Work out the finished part from the listing and answer in its coordinate system (mm). A direction names the side the tool comes from. Give positions to 0.01 mm unless a question says otherwise; leave off trailing zeros. Loops run counter-clockwise (first coordinate to the right, second up) from the corner with the lowest first, then second, coordinate; pieces in that order, holes last. Notation, with made-up numbers: (83.25, -32) - (112.25, -32) arc R31 ccw to (112.25, 5) - close; hole circle Ø5 at (-10, 59). An arc over 180 degrees is marked (long way). One line per question, with ' | ' between items.
from build123d import *

# Parameters (mm, degrees)
SKIZZE1_W                                  = 70
SKIZZE1_H                                  = 20
AUFSATZ_LINEAR_AUSTRAGEN1_DEPTH            = 20
F_5_2_5_2_DURCHMESSER_BOHRUNG1_D           = 5.2
F_5_2_5_2_DURCHMESSER_BOHRUNG1_CSINK_D     = 5.25
F_5_2_5_2_DURCHMESSER_BOHRUNG1_CSINK_ANGLE = 90
SKIZZE21_R                                 = 6.05
SCHNITT_LINEAR_AUSTRAGEN3_DEPTH            = 7
SKIZZE22_R                                 = 4
SCHNITT_LINEAR_AUSTRAGEN5_DEPTH            = 10


# Read off the part's stored shape, not the designer's step: Durchgangsloch für M3.51
with BuildPart() as part:
    # Skizze1 → Aufsatz-Linear austragen1 (new body)
    with BuildSketch(Plane.XY):
        with Locations((0, 1.677024639)):
            Rectangle(SKIZZE1_W, SKIZZE1_H)
    extrude(amount=AUFSATZ_LINEAR_AUSTRAGEN1_DEPTH)

    # Ø5.2 (5.2) Durchmesser Bohrung1 (through all)
    with Locations(Plane.XY.offset(20)):
        with Locations((-28, 0.177024639), (28, 0.177024639)):
            CounterSinkHole(F_5_2_5_2_DURCHMESSER_BOHRUNG1_D / 2, F_5_2_5_2_DURCHMESSER_BOHRUNG1_CSINK_D / 2, counter_sink_angle=F_5_2_5_2_DURCHMESSER_BOHRUNG1_CSINK_ANGLE)

    # Durchgangsloch für M3.51 outline → Durchgangsloch für M3.51 (revolve, cut)
    with BuildSketch(Plane(origin=(-28, 0, 10), x_dir=(1, 0, 0), z_dir=(0, 0, 1))):
        Polygon((1.85, -8.297975361), (1.85, -1.649435315), (0, -1.649435315), (0, -8.322975361), (1.875, -8.322975361), align=None)
    revolve(axis=Axis((-28, 0, 10), (0, 1, 0)), mode=Mode.SUBTRACT)

    # Durchgangsloch f_r M3.51 2 outline → Durchgangsloch f_r M3.51 2 (revolve, cut)
    with BuildSketch(Plane(origin=(28, 0, 10), x_dir=(1, 0, 0), z_dir=(0, 0, 1))):
        Polygon((1.85, -8.297975361), (1.85, -1.649435315), (0, -1.649435315), (0, -8.322975361), (1.875, -8.322975361), align=None)
    revolve(axis=Axis((28, 0, 10), (0, 1, 0)), mode=Mode.SUBTRACT)

    # Skizze21 → Schnitt-Linear austragen3 (cut)
    with BuildSketch(Plane(origin=(0, 0, 0), x_dir=(-1, 0, 0), z_dir=(0, 0, -1))):
        Circle(SKIZZE21_R)
    extrude(amount=-SCHNITT_LINEAR_AUSTRAGEN3_DEPTH, mode=Mode.SUBTRACT)

    # Skizze22 → Schnitt-Linear austragen5 (cut)
    with BuildSketch(Plane(origin=(0, 0, 7), x_dir=(-1, 0, 0), z_dir=(0, 0, -1))):
        Circle(SKIZZE22_R)
    extrude(amount=-SCHNITT_LINEAR_AUSTRAGEN5_DEPTH, mode=Mode.SUBTRACT)


solid = part.part
1. Find section A-A on x = 28. Write down the section's boundary in (y, z) (3 decimals).
Evaluation:
outline: (-8.323, 0) - (-2.423, 0) - (-2.423, 8.15) - (-8.298, 8.15) - (-8.323, 8.125) - close; (-8.323, 11.875) - (-8.298, 11.85) - (-2.423, 11.85) - (-2.423, 19.975) - (-2.448, 20) - (-8.323, 20) - close; (2.777, 0) - (11.677, 0) - (11.677, 20) - (2.802, 20) - (2.777, 19.975) - close
2. Which of the six approach directions +Z, -Z, +X, -X, +Y, -Y give full straight-line access (tool end or side, diameter ignored) to faces 4 (the flat face through (1.43, -3.95, 7)), 5 (the cylindrical face through (-28.401, -4.927, 11.806)), 6 (the flat face through (0, 11.677, 10))?
Evaluation:
face 4: -Z | face 5: -Y | face 6: +Z, -Z, +X, -X, +Y
3. Consider L1, parallel to Z at x = -28, y = -5.25; L2, parallel to X at y = -2.75, z = 10; L3, parallel to X at y = -2, z = 16.25. Determine where each line is inside the solid, lowest interval first.
Evaluation:
L1: 0 to 8.15, 11.85 to 20 | L2: -35 to -29.85, -26.15 to -2.9, 2.9 to 26.15, 29.85 to 35 | L3: -35 to -29.42, -26.58 to -3.46, 3.46 to 26.58, 29.42 to 35
4. Determine the mould class of faces 1 (the cylindrical face through (27.599, -4.927, 11.806)), 2 (the flat face through (0, 2, 20)), 3 (the flat face through (-35, 2, 10)) for opening direction Z: +Z half, -Z half, draft (parallel to the pull), parting line (faces both ways), or undercut.
Evaluation:
face 1: undercut | face 2: +Z half | face 3: draft
5. Find section B-B on z = 10. Write down the section's boundary in (x, y) (3 decimals).
Evaluation:
outline: (-35, -8.323) - (-29.875, -8.323) - (-29.85, -8.298) - (-29.85, -1.65) arc R2.6 cw (long way) to (-26.15, -1.65) - (-26.15, -8.298) - (-26.125, -8.323) - (26.125, -8.323) - (26.15, -8.298) - (26.15, -1.65) arc R2.6 cw (long way) to (29.85, -1.65) - (29.85, -8.298) - (29.875, -8.323) - (35, -8.323) - (35, 11.677) - (-35, 11.677) - close; hole circle Ø8 at (0, 0)
6. Find section C-C on x = 0. Write down the section's boundary in (y, z).
Evaluation:
outline: (-8.32, 0) - (-6.05, 0) - (-6.05, 7) - (-4, 7) - (-4, 17) - (4, 17) - (4, 7) - (6.05, 7) - (6.05, 0) - (11.68, 0) - (11.68, 20) - (-8.32, 20) - close
7. Find section D-D on y = -5.25. Write down the section's boundary in (x, z).
Evaluation:
outline: (-35, 0) - (-3.01, 0) - (-3.01, 7) - (3.01, 7) - (3.01, 0) - (35, 0) - (35, 20) - (-35, 20) - close; hole circle Ø3.7 at (-28, 10); hole circle Ø3.7 at (28, 10)
8. Flat-ended cylindrical pins translate along their axes: pin 1 (2 mm diameter, centred on x = 11, y = -0.5, fed in from -Z); pin 2 (4 mm diameter, centred on x = -28, y = 0.18, fed in from -Z); pin 3 (7 mm diameter, centred on x = 0, y = 0, fed in from -Z). Find the tip coordinate at first contact, or state that the pin passes through.
Evaluation:
pin 1: z = 0 | pin 2: through | pin 3: z = 17
